CAD build for the part. Positions are in the model's coordinates, mm. Round coordinates to 2 decimals unless told otherwise and drop trailing zeros. Loops run counter-clockwise (first coordinate to the right, second up) from the corner with the lowest first, then second, coordinate; pieces in that order, holes last.
```python
from build123d import *

# Parameters (mm, degrees)
F0_R            = 67.5
F0_R_2          = 5
F1_DEPTH        = 5
F3_D            = 12
F3_COPIES_COUNT = 3


# Not quite as in the source:
# - a pattern or mirror of a feature is missing from the dataset's text; its kind, count and spacing are read off the source's solid


with BuildPart() as f1:
    # F0 (on Top) → F1 (new body)
    with BuildSketch(Plane.XY):
        Circle(F0_R)
        Circle(F0_R_2, mode=Mode.SUBTRACT)
    extrude(amount=F1_DEPTH)

    # F3 (through all)
    with Locations(Plane.XY.offset(5)):
        with Locations((54, 0)):
            f3 = Hole(F3_D / 2)

    # F3_copies: F3 ×3 about axis
    f3_copies_axis = Axis((0, 0, 0), (0, 0, 1))
    for i in range(1, F3_COPIES_COUNT):
        add(f3.rotate(f3_copies_axis, i * 360 / F3_COPIES_COUNT), mode=Mode.SUBTRACT)


solid = f1.part
```
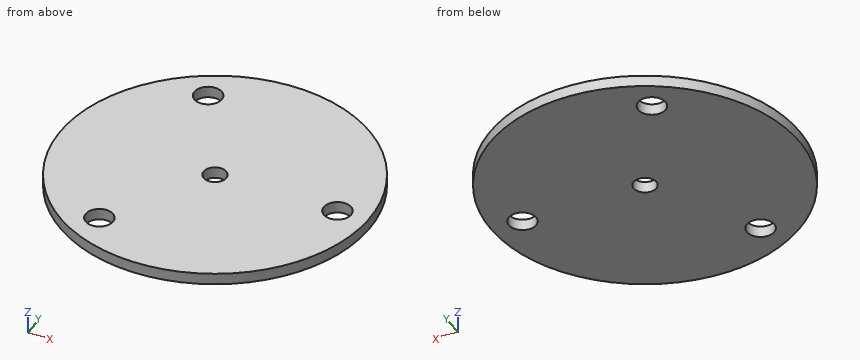
Item 1: Probe line 1 (Y direction, x = 0, z = 3.35); line 2 (Y direction, x = -27, z = 2.35); line 3 (X direction, y = -51, z = 2.95). List the from-to ranges inside material, lowest first.
Answers follow:
line 1: y = -67.5 to -5, 5 to 67.5
line 2: y = -61.86 to -52.77, -40.77 to 40.77, 52.77 to 61.86
line 3: x = -44.22 to -31.25, -22.75 to 44.22
Item 2: Cut at B-B, the plane y = 0. Give the cut face in (x, z), plus the area to 3 significant figures.
Answers follow:
outline: (-67.5, 0) - (-5, 0) - (-5, 5) - (-67.5, 5) - close; (5, 0) - (48, 0) - (48, 5) - (5, 5) - close; (60, 0) - (67.5, 0) - (67.5, 5) - (60, 5) - close
area: 565 mm2
Item 3: Cut at A-A, the plane x = 0. Give the cut face in (y, z), plus the area to 3 significant figures.
Answers follow:
outline: (-67.5, 0) - (-5, 0) - (-5, 5) - (-67.5, 5) - close; (5, 0) - (67.5, 0) - (67.5, 5) - (5, 5) - close
area: 625 mm2
Item 4: Flat gauge pins, fed straight in: P1, Ø3, axis at y = -37, z = 2.5, coming from the +X side; P2, Ø1.5, axis at y = -14, z = 3, coming from the -X side; P3, Ø1, axis at y = -26, z = 3, coming from the -X side. Where does each tip first touch, or does it go through?
Answers follow:
P1: stops at x = 57.41
P2: stops at x = -66.19
P3: stops at x = -62.5
Item 5: Cut at C-C, the plane x = -27. Give the cut face in (y, z).
Answers follow:
outline: (-61.86, 0) - (-52.77, 0) - (-52.77, 5) - (-61.86, 5) - close; (-40.77, 0) - (40.77, 0) - (40.77, 5) - (-40.77, 5) - close; (52.77, 0) - (61.86, 0) - (61.86, 5) - (52.77, 5) - close
Item 6: Cut at D-D, the plane y = -49.5. Give the cut face in (x, z), plus the area to 3 significant figures.
Answers follow:
outline: (-45.89, 0) - (-32.34, 0) - (-32.34, 5) - (-45.89, 5) - close; (-21.66, 0) - (45.89, 0) - (45.89, 5) - (-21.66, 5) - close
area: 406 mm2
